Source: three-view drawing plus pictorial views. Frame: mm from the lowest corner of the part. A direction names the side the tool comes from. Coordinates: 2 decimals unless noted, no trailing zeros. Write each loop counter-clockwise with the first axis right and the second up, starting at its lowest first coordinate (ties: lowest second). Pieces come first, ordered by that corner, then holes. Notation, with made-up numbers: (3.25, -10.5) - (8.25, -10.5) arc R34 cw to (8.25, 20.5) - close; hole circle Ø8 at (-17, -26). An arc over 180 degrees is marked (long way). Put each result on its own line as item: value. Start each with the question number.
1. Line query: line 1 (Y direction, x = 15, z = 10); line 2 (X direction, y = 3.65, z = 7.5); line 3 (X direction, y = 20.75, z = 10). Output: solid intervals per line, ascending.
2. Pin query (flat end, axial travel): pin 1 (6 mm diameter, centred on y = 13, z = 12.5, fed in from +X); pin 2 (3 mm diameter, centred on x = 66, y = 5, fed in from +Z); pin 3 (3 mm diameter, centred on x = 3, z = 9.5, fed in from +Y); pin 4 (4.5 mm diameter, centred on x = 49.5, z = 8.5, fed in from -Y). Return the tip coordinate at first contact, or that it passes through.
3. Cut plane B-B, the plane x = 66. Return loops of the section in (y, z), and give its area (3 significant figures).
4. Cut plane A-A, the plane y = 9.75. Return loops of the section in (x, z), and give its area (3 significant figures).
5. Access query for the marked faces 1, 2, 3 and 4. Directions: +Z, -Z, +X, -X, +Y, -Y. A direction counts if a zero-diameter tool reaches every point of the face in a straight line with its end or side. Return the directions, or none.
6. Pull-direction query (X, two-part tool) for the marked faces 5, 6 and 7; classes: released by +X, released by -X, zero draft, split by the parting line, or undercut.
7. Cut plane D-D, the plane x = 76. Return loops of the section in (y, z).
8. Cut plane C-C, the plane z = 6.75. Return loops of the section in (x, y).
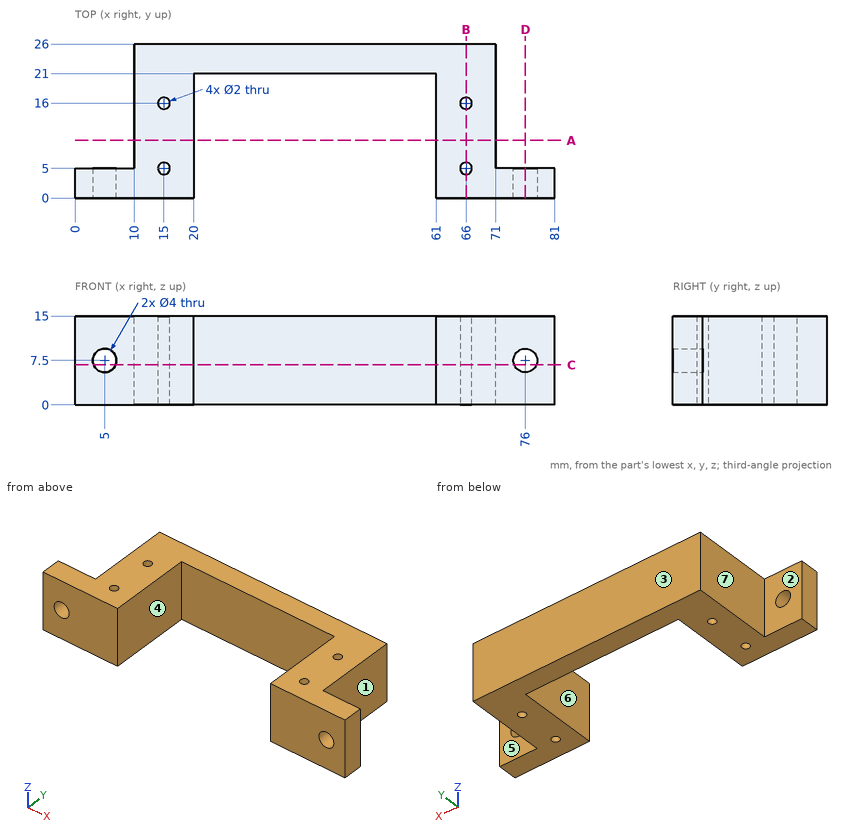
Report:
1. line 1: y = 0 to 4, 6 to 15, 17 to 26
1. line 2: x = 0 to 3, 7 to 20, 61 to 74, 78 to 81
1. line 3: x = 10 to 20, 61 to 71
2. pin 1: stops at x = 71
2. pin 2: stops at z = 15
2. pin 3: stops at y = 5
2. pin 4: stops at y = 21
3. outline: (0, 0) - (4, 0) - (4, 15) - (0, 15) - close; (6, 0) - (15, 0) - (15, 15) - (6, 15) - close; (17, 0) - (26, 0) - (26, 15) - (17, 15) - close
3. area: 330 mm^2
4. outline: (10, 0) - (20, 0) - (20, 15) - (10, 15) - close; (61, 0) - (71, 0) - (71, 15) - (61, 15) - close
4. area: 300 mm^2
5. face 1: +Z, -Z, +X, +Y
5. face 2: +Z, -Z, -X, +Y
5. face 3: +Z, -Z, +X, -X, +Y
5. face 4: +Z, -Z, -Y
6. face 5: zero draft
6. face 6: undercut
6. face 7: released by -X
7. outline: (0, 0) - (5, 0) - (5, 5.5) - (0, 5.5) - close; (0, 9.5) - (5, 9.5) - (5, 15) - (0, 15) - close
8. outline: (0, 0) - (3.15, 0) - (3.15, 5) - (0, 5) - close; (6.85, 0) - (20, 0) - (20, 21) - (61, 21) - (61, 0) - (74.15, 0) - (74.15, 5) - (71, 5) - (71, 26) - (10, 26) - (10, 5) - (6.85, 5) - close; (77.85, 0) - (81, 0) - (81, 5) - (77.85, 5) - close; hole circle Ø2 at (15, 5); hole circle Ø2 at (15, 16); hole circle Ø2 at (66, 5); hole circle Ø2 at (66, 16)
